Answer from the drawing. Dimensions are ordinates in mm from the lowest x, y and z of the part. Coordinates: 2 decimals unless noted, no trailing zeros. Order: outer loops, then holes, each group sorted by start corner. A loop starts at its lowest first (then second) coordinate and runs counter-clockwise, first axis right, second up. Notation, with made-up numbers: (7, 32.5) -> (17, 32.5) arc R28 ccw to (17, 70.5) -> close; hole circle Ø9 at (-27, 52.25). An arc over 180 degrees is marked (long way). Answer in a Markdown table with one row per item.
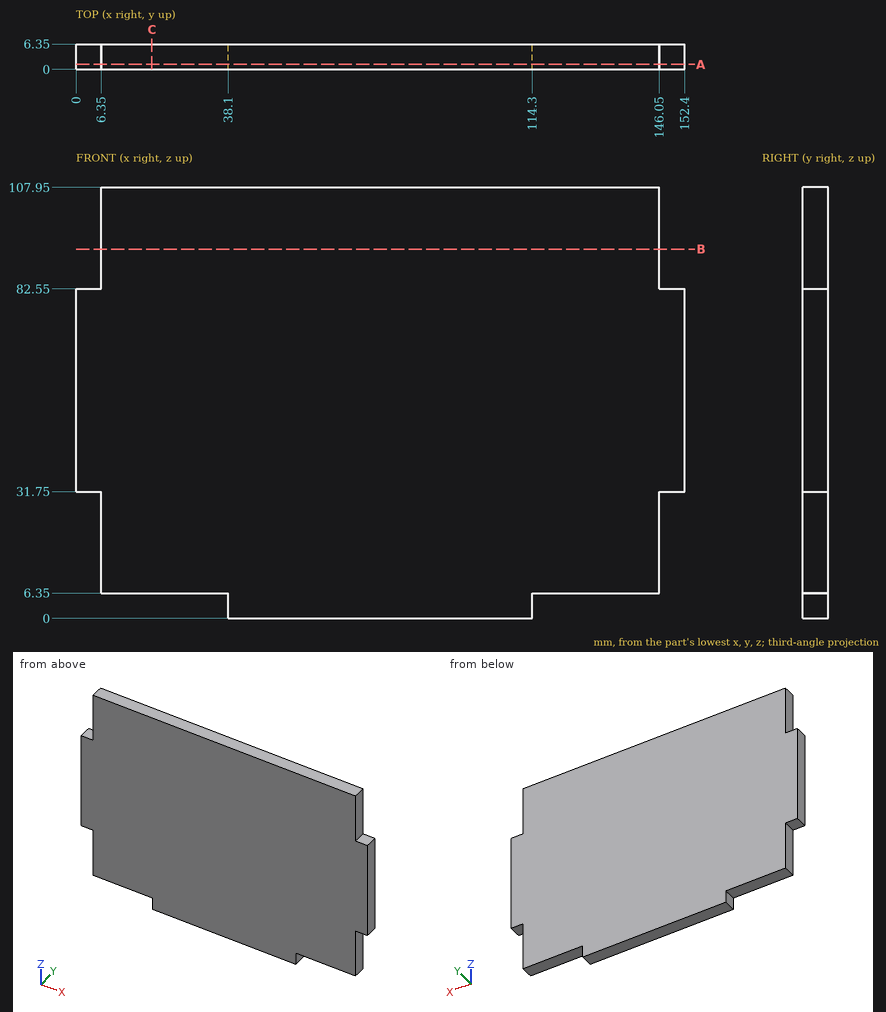
Q1. The part is cut by section B-B (z = 92.5). Write down the section's boundary in (x, y), then the cut area to 3 significant figures.
Outcome:
| item | result |
|---|---|
| outline | (6.35, 0) -> (146.05, 0) -> (146.05, 6.35) -> (6.35, 6.35) -> close |
| area | 887 mm² |
Q2. The part is cut by section C-C (x = 19). Write down the section's boundary in (y, z), then the cut area to 3 significant figures.
Outcome:
| item | result |
|---|---|
| outline | (0, 6.35) -> (6.35, 6.35) -> (6.35, 107.95) -> (0, 107.95) -> close |
| area | 645 mm² |
Q3. Consider line 1 (Z direction, x = 129, y = 2); line 2 (X direction, y = 6, z = 10.5). Determine where each line is inside the solid, lowest interval first.
Outcome:
| item | result |
|---|---|
| line 1 | 6.35 to 107.95 |
| line 2 | 6.35 to 146.05 |
Q4. The part is cut by section A-A (y = 1.25). Write down the section's boundary in (x, z), then the cut area to 3 significant figures.
Outcome:
| item | result |
|---|---|
| outline | (0, 31.75) -> (6.35, 31.75) -> (6.35, 6.35) -> (38.1, 6.35) -> (38.1, 0) -> (114.3, 0) -> (114.3, 6.35) -> (146.05, 6.35) -> (146.05, 31.75) -> (152.4, 31.75) -> (152.4, 82.55) -> (146.05, 82.55) -> (146.05, 107.95) -> (6.35, 107.95) -> (6.35, 82.55) -> (0, 82.55) -> close |
| area | 15,300 mm² |
Q5. Given pin 1 (1.9 mm diameter, centred on x = 148.5, y = 3, fed in from -Z); pin 2 (1.9 mm diameter, centred on x = 15, y = 3, fed in from -Z); pin 3 (1.9 mm diameter, centred on y = 2.5, z = 14.5, fed in from -X); pin 4 (2 mm diameter, centred on x = 77.5, z = 55, fed in from -Y), each flat-ended and moving along its own axis, determine where each tip first touches the part or whether it passes through.
Outcome:
| item | result |
|---|---|
| pin 1 | z = 31.75 |
| pin 2 | z = 6.35 |
| pin 3 | x = 6.35 |
| pin 4 | y = 0 |
